For this review, take the finished solid that the model builds, in its own axes (mm). A direction names the side the tool comes from. Give positions to 0.01 mm unless a question says otherwise; leave off trailing zeros. Loops run counter-clockwise (first coordinate to the right, second up) from the corner with the lowest first, then second, coordinate; pieces in that order, holes last. Notation, with made-up numbers: (13.25, -5) -> (19.25, -5) arc R25 cw to (19.25, 33) -> close; hole circle Ø9 at (32, -16). An arc over 180 degrees is marked (long way). One line per question, with ' | ' between items. Start each with the question number.
(1) Wall thickness on probe 1 along Y at (x, z) = (0, 23.45); probe 2 along X at (y, z) = (-8.75, -0.5); probe 3 along Y at (x, z) = (3.5, -3.5): over which ranges is each line inside the solid? List them lowest first.
(2) Tool access review of faces 1 (the flat face through (0, -12.25, 9)), 2 (the flat face through (-4.05, 0, -3)): name each direction out of +Z, -Z, +X, -X, +Y, -Y from which nothing blocks a thin tool from reaching the whole face with its end or side.
(3) Consider section C-C (z = 11.5). Write out the cut boundary in (x, y), and give its area (3 significant figures).
(4) Insertion check: P1, Ø5, axis at x = 0, y = -5.46, coming from the -Z side; P2, Ø2, axis at x = -3.5, y = -6.5, coming from the +Z side; P3, Ø1.5, axis at x = 2.5, y = -1, coming from the -Z side; P4, Ø4, axis at x = 0, y = -5.46, coming from the +Z side. Each pin has a flat end and moves straight along its axis. Give the tip position at first contact, or say it passes through.
(5) Draft analysis for pull direction Z (two halves, no side actions). For faces 3 (the cylindrical face through (2.956, -6.688, 16.031)), 4 (the flat face through (0, 0, 25)), 5 (the flat face through (0, 3, 0)), 6 (the cylindrical face through (-0.49, -7.66, 5.93)), state which applies: +Z half, -Z half, draft (parallel to the pull), parting line (faces both ways), or undercut.
(6) Consider section A-A (z = 6.5). Write out the cut boundary in (x, y), and give its area (3 significant figures).
(7) Consider section B-B (y = 0). Write out the cut boundary in (x, z), and give its area (3 significant figures).
from build123d import *

# Parameters (mm, degrees)
F0_W         = 11.3
F0_H         = 24.5
F0_W_2       = 8.1
F0_H_2       = 21.3
F1_DEPTH     = 1
F2_DEPTH     = 6
F3_R         = 3.2
F4_DEPTH     = 24
F5_DEPTH     = 28.9
F8_R         = 0.5
F9_SIZE      = 0.5
F10_R        = 3.2
F10_R_2      = 2.25
F11_DEPTH    = 12
F12_S5_R     = 3.2
F12_T6_DEPTH = 6
F13_SIZE     = 1


# Not quite as in the source:
# - a fillet or chamfer that OpenCascade refuses, or shapes differently, is made with other operations: its cross-section is extruded or revolved along the edge and cut away or added


with BuildPart() as f1:
    # F0 (on Top) → F1 (new body)
    with BuildSketch(Plane.XY):
        Rectangle(F0_W, F0_H)
        Rectangle(F0_W_2, F0_H_2, mode=Mode.SUBTRACT)
        Rectangle(F0_W_2, F0_H_2)
    extrude(amount=F1_DEPTH)

    # F0 (on Top) → F2 (join)
    with BuildSketch(Plane.XY):
        Rectangle(F0_W, F0_H)
        Rectangle(F0_W_2, F0_H_2, mode=Mode.SUBTRACT)
    extrude(amount=-F2_DEPTH)

    # F3 (on face) → F4 (join)
    with BuildSketch(Plane.XY.offset(1)):
        with BuildLine():
            ThreePointArc((-5.65, -5.4622520893), (1e-08, -11.1122520693), (5.65, -5.4622520693))
            ThreePointArc((5.65, -5.4622520693), (-1e-08, 0.1877479307), (-5.65, -5.4622520893))
        make_face()
        with Locations((0, -5.4622520693)):
            Circle(F3_R, mode=Mode.SUBTRACT)
        with BuildLine():
            Line((5.65, -12.25), (5.65, -5.4622520693))
            ThreePointArc((5.65, -5.4622520693), (1e-08, -11.1122520693), (-5.65, -5.4622520893))
            Line((-5.65, -5.4622520893), (-5.65, -12.25))
            Line((-5.65, -12.25), (5.65, -12.25))
        make_face()
        with BuildLine():
            ThreePointArc((-5.65, -5.4622520893), (-1e-08, 0.1877479307), (5.65, -5.4622520693))
            Line((5.65, -5.4622520693), (5.65, 12.25))
            Line((5.65, 12.25), (-5.65, 12.25))
            Line((-5.65, 12.25), (-5.65, -5.4622520893))
        make_face()
    extrude(amount=F4_DEPTH)

    # F5 (cut): a face of the model
    f5_faces = [f1.faces().sort_by_distance(p)[0] for p in [
        (0, -5.4622520693, 1),
    ]]
    extrude(f5_faces, amount=-F5_DEPTH, mode=Mode.SUBTRACT)

    # F6 (on Right) → F7 (revolve)
    with BuildSketch(Plane.YZ):
        Polygon((-8.6622520693, 22), (-8.6622520693, 20), (-7.6622520693, 21), align=None)
    revolve(axis=Axis((0, -5.4622520693, 1), (0, 0, -1)))

    # F8
    f8_edges = [f1.edges().sort_by_distance(p)[0] for p in [
        (0, -3.262252, 21),
    ]]
    fillet(f8_edges, radius=F8_R)

    # F9
    f9_edges = [f1.edges().sort_by_distance(p)[0] for p in [
        (-5.65, 0, 25),
        (0, -12.25, 25),
        (5.65, 0, 25),
        (0, 12.25, 25),
        (-3.2, -5.462252, 25),
    ]]
    chamfer(f9_edges, length=F9_SIZE)

    # F10 (on face) → F11 (join)
    with BuildSketch(Plane.XY):
        with Locations((0, -5.4622520693)):
            Circle(F10_R)
        with Locations((0, -5.4622520693)):
            Circle(F10_R_2, mode=Mode.SUBTRACT)
    extrude(amount=F11_DEPTH)

    # F12: chamfer of 1 on 1 edges, made by hand


with BuildPart() as f12_tool2:
    # F12_s3 → F12_t4 (revolve)
    with BuildSketch(Plane.XZ.offset(5.4622520693)):
        Polygon((3.25, 12), (2.25, 11), (2.25, 12), align=None)
    revolve(axis=Axis((0, -5.4622520693, 12), (0, 0, 1)))

    # F12_s5 → F12_t6 (intersect, symmetric)
    with BuildSketch(Plane.XY.offset(11.5)):
        with Locations((0, -5.4622520693)):
            Circle(F12_S5_R)
    extrude(amount=F12_T6_DEPTH, both=True, mode=Mode.INTERSECT)


with BuildPart() as f1_1:
    add(f1.part)

    # F12_t1: cut F12_tool2
    add(f12_tool2.part, mode=Mode.SUBTRACT)

    # F13
    f13_edges = [f1_1.edges().sort_by_distance(p)[0] for p in [
        (-2.25, -5.462252, 0),
    ]]
    chamfer(f13_edges, length=F13_SIZE)


solid = f1_1.part
A:
1) probe 1: y = -12.25 to -8.66, -2.26 to 12.25 | probe 2: x = -5.65 to -4.05, 4.05 to 5.65 | probe 3: y = -12.25 to -10.65, 10.65 to 12.25
2) face 1: +Z, -Z, +X, -X, -Y | face 2: -Z
3) outline: (-5.65, -12.25) -> (5.65, -12.25) -> (5.65, 12.25) -> (-5.65, 12.25) -> close; hole circle Ø5.5 at (0, -5.46) | area: 253 mm^2
4) P1: stops at z = 0.75 | P2: stops at z = 25 | P3: stops at z = 0 | P4: passes through
5) face 3: undercut | face 4: +Z half | face 5: -Z half | face 6: draft
6) outline: (-5.65, -12.25) -> (5.65, -12.25) -> (5.65, 12.25) -> (-5.65, 12.25) -> close; hole circle Ø4.5 at (0, -5.46) | area: 261 mm^2
7) outline: (-5.65, -6) -> (-4.05, -6) -> (-4.05, 0) -> (4.05, 0) -> (4.05, -6) -> (5.65, -6) -> (5.65, 24.5) -> (5.15, 25) -> (-5.15, 25) -> (-5.65, 24.5) -> close | area: 301 mm^2
